```python
from build123d import *

# Parameters (mm, degrees)
SKETCH_1_R                   = 75
SKETCH_1_R_2                 = 17.25
EXTRUDE_1_DEPTH              = 5
EXTRUDE_START                = -5
SKETCH_2_R                   = 17.25
EXTRUDE_2_DEPTH              = 5
HOLE_WIZARD_M4_5_D           = 3.3
HOLE_WIZARD_M4_5_CSINK_D     = 4.05
HOLE_WIZARD_M4_5_CSINK_ANGLE = 90
PATTERN_CIRCULAR_1_COUNT     = 6


with BuildPart() as part:
    # 草图1 → 凸台-拉伸1 (new body)
    with BuildSketch(Plane.XY):
        with Locations((-61.833180774, 36.701596564)):
            Circle(SKETCH_1_R)
        with Locations((-61.833180774, 36.701596564)):
            Circle(SKETCH_1_R_2, mode=Mode.SUBTRACT)
    extrude(amount=EXTRUDE_1_DEPTH)

    # 草图2 → 凸台-拉伸2 (add)
    with BuildSketch(Plane.XY.offset(5).offset(EXTRUDE_START)):
        with Locations((-61.833180774, 36.701596564)):
            Circle(SKETCH_2_R)
    extrude(amount=EXTRUDE_2_DEPTH)

    # M4 螺纹孔5 (through all)
    with Locations(Plane.XY.offset(5)):
        with Locations((-79.083180774, 36.701596564)):
            hole_wizard_m4_5 = CounterSinkHole(HOLE_WIZARD_M4_5_D / 2, HOLE_WIZARD_M4_5_CSINK_D / 2, counter_sink_angle=HOLE_WIZARD_M4_5_CSINK_ANGLE)

    # 阵列(圆周)1: M4 螺纹孔5 ×6 about axis
    pattern_circular_1_axis = Axis((-61.833180774, 36.701596564, 0), (0, 0, 1))
    for i in range(1, PATTERN_CIRCULAR_1_COUNT):
        add(hole_wizard_m4_5.rotate(pattern_circular_1_axis, i * 360 / PATTERN_CIRCULAR_1_COUNT), mode=Mode.SUBTRACT)


solid = part.part
```
Design review of the part built by this model. Coordinates are the model's own, in mm. Coordinates: 2 decimals unless noted, no trailing zeros. Write each loop counter-clockwise with the first axis right and the second up, starting at its lowest first coordinate (ties: lowest second). Pieces come first, ordered by that corner, then holes.
1) Add section C-C (y = 71.5). Write out the cut boundary in (x, z), plus the area to 3 significant figures.
2) Add section B-B (x = -117). Write out the cut boundary in (y, z), plus the area to 3 significant figures.
3) Mouldability with a two-part tool opening along Y and no side actions: class faces 1 (the flat face through (-63, 38, 5)), 2 (the cylindrical face through (7.45, 7.98, 2.46)), 3 (the cylindrical face through (-51.992, 52.756, 2.28)) as +Y half, -Y half, draft (parallel to the pull), parting line (faces both ways), or undercut.
4) Add section A-A (z = 3). Write out the cut boundary in (x, y).
5) Insertion check: pin 1 (2.5 mm diameter, centred on x = -53.21, y = 51.64, fed in from +Z); pin 2 (1.5 mm diameter, centred on y = -3.5, z = 3.5, fed in from +X); pin 3 (1.5 mm diameter, centred on y = 2, z = 2, fed in from +X); pin 4 (1 mm diameter, centred on y = 16, z = 1.5, fed in from -X). Each pin has a flat end and moves straight along its axis. Give the tip position at first contact, or say it passes through.
6) To check wall thickness, follow L1, parallel to Y at x = -54, z = 1; L2, parallel to X at y = 52, z = 0.5; L3, parallel to Y at x = -78.5, z = 3.3. State the ranges of each line that lie inside material, in increasing order.
Check result:
1. outline: (-128.27, 0) - (4.61, 0) - (4.61, 5) - (-128.27, 5) - close
1. area: 664 mm2
2. outline: (-14.11, 0) - (87.51, 0) - (87.51, 5) - (-14.11, 5) - close
2. area: 508 mm2
3. face 1: draft
3. face 2: parting line
3. face 3: undercut
4. outline: circle Ø150 at (-61.83, 36.7); hole circle Ø3.3 at (-79.08, 36.7); hole circle Ø3.3 at (-70.46, 21.76); hole circle Ø3.3 at (-70.46, 51.64); hole circle Ø3.3 at (-53.21, 21.76); hole circle Ø3.3 at (-53.21, 51.64); hole circle Ø3.3 at (-44.58, 36.7)
5. pin 1: passes through
5. pin 2: stops at x = 1.95
5. pin 3: stops at x = 5.04
5. pin 4: stops at x = -134.06
6. L1: y = -37.89 to 20.32, 23.21 to 50.19, 53.09 to 111.29
6. L2: x = -135.26 to -72.07, -68.85 to -54.82, -51.6 to 11.59
6. L3: y = -36.42 to 35.16, 38.25 to 109.83
